from build123d import *


with BuildPart() as part:
    # Táhnout po křivce1: sweep along a path in Skica4
    with BuildLine(Plane(origin=(0, 0, 0), x_dir=(0, 0, -1), z_dir=(1, 0, 0))) as t_hnout_po_k_ivce1_path:
        Line((0, 0), (0, 90))
        ThreePointArc((0, 90), (-2.928932188, 97.071067812), (-10, 100))
        Line((-10, 100), (-25, 100))
    # Skica2 → Táhnout po křivce1 (sweep)
    with BuildSketch(Plane(origin=(0, 0, 0), x_dir=(1, 0, 0), z_dir=(0, 1, 0))):
        Polygon((2.309401077, -4), (4.618802154, 0), (2.309401077, 4), (-2.309401077, 4), (-4.618802154, 0), (-2.309401077, -4), align=None)
    sweep(path=t_hnout_po_k_ivce1_path.line)


solid = part.part
Geometry: final body of the model. Coordinates: model frame, mm. A direction names the side the tool comes from. Round coordinates to 2 decimals unless told otherwise and drop trailing zeros. Order: outer loops, then holes, each group sorted by start corner. A loop starts at its lowest first (then second) coordinate and runs counter-clockwise, first axis right, second up.
Q1. Section B-B, the plane z = 12.5. Output: boundary loops of the cut face in (x, y).
Result sheet:
outline: (-4.62, 100) - (-2.31, 96) - (2.31, 96) - (4.62, 100) - (2.31, 104) - (-2.31, 104) - close
Q2. Material intervals for probe 1 along Z at (x, y) = (0, 49); probe 2 along Z at (x, y) = (4, 7); probe 3 along Y at (x, z) = (-3, 17.75), sorted ascending.
Result sheet:
probe 1: z = -4 to 4
probe 2: z = -1.07 to 1.07
probe 3: y = 97.2 to 102.8
Q3. Section D-D, the plane x = 3.75. Output: boundary loops of the cut face in (y, z), and give its area (3 significant figures).
Result sheet:
outline: (0, -1.5) - (90, -1.5) arc R11.5 ccw to (101.5, 10) - (101.5, 25) - (98.5, 25) - (98.5, 10) arc R8.5 cw to (90, 1.5) - (0, 1.5) - close
area: 363 mm2
Q4. Section A-A, the plane x = -0.25. Output: boundary loops of the cut face in (y, z), and give its area (3 significant figures).
Result sheet:
outline: (0, -4) - (90, -4) arc R14 ccw to (104, 10) - (104, 25) - (96, 25) - (96, 10) arc R6 cw to (90, 4) - (0, 4) - close
area: 966 mm2
Q5. Pin query (flat end, axial travel): pin 1 (5 mm diameter, centred on x = 0, y = 61.5, fed in from +Z); pin 2 (4 mm diameter, centred on x = -2, z = 5.5, fed in from +Y) (3 decimals); pin 3 (4 mm diameter, centred on y = 58, z = 7.5, fed in from +X) (3 decimals); pin 4 (6 mm diameter, centred on y = 10.5, z = 6, fed in from -X). Return the tip coordinate at first contact, or that it passes through.
Result sheet:
pin 1: stops at z = 4
pin 2: stops at y = 103.775
pin 3: passes through
pin 4: stops at x = -2.89
Q6. Access query for faces 1 (the face through (0, 96, 18)), 2 (the face through (-3.48, 45.63, 1.97)), 3 (the face through (3.48, 101.97, 17.61)), 4 (the face through (-3.448, 102.028, 17.605)), 5 (the face through (3.448, 97.972, 17.605)). Directions: +Z, -Z, +X, -X, +Y, -Y. A direction counts if a zero-diameter tool reaches every point of the face in a straight line with its end or side. Return the directions, or none.
Result sheet:
face 1: +Z, +X, -X, -Y
face 2: +Z, -X, -Y
face 3: +Z, -Z, +X, +Y
face 4: +Z, -Z, -X, +Y
face 5: +Z, +X, -Y
Q7. Section C-C, the plane y = 79.5. Output: boundary loops of the cut face in (x, z), and give its area (3 significant figures).
Result sheet:
outline: (-4.62, 0) - (-2.31, -4) - (2.31, -4) - (4.62, 0) - (2.31, 4) - (-2.31, 4) - close
area: 55.4 mm2
